Work out the finished part from the listing and answer in its coordinate system (mm). Give positions to 0.01 mm unless a question says otherwise; leave off trailing zeros. Order: outer loops, then holes, each group sorted by start corner. A loop starts at its lowest first (then second) coordinate and runs counter-clockwise, first axis right, second up. Notation, with made-up numbers: (77, 75.25) - (88, 75.25) arc R20 cw to (88, 113.25) - close; hole circle Ø1 at (-2, -12). An arc over 180 degrees is marked (long way). Write each question's results on one line, items separated by ' | '.
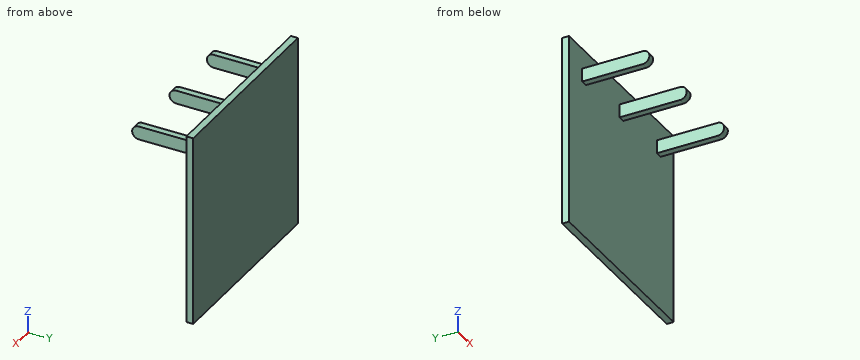
Autodesk Inventor part; units mm, degrees
ref_plane "pole_to_body_XY" through (0, 0.508, 0) normal (0, 1, 0) x (1, 0, 0)
ref_plane "pole_to_body_YZ" through (0, 0.508, 0) normal (1, 0, 0) x (0, 0, -1)
ref_plane "pole_to_body_ZX" through (0, 0.508, 0) normal (0, 0, -1) x (0, 1, 0)
sketch "Sketch_1" plane through (0, 0, 0) normal (0, 1, 0) x (-1, 0, 0)
  line L0 (7.112, -7.112) -> (7.112, 7.112)
  line L1 (7.112, 7.112) -> (-7.112, 7.112)
  line L2 (-7.112, 7.112) -> (-7.112, -7.112)
  line L3 (-7.112, -7.112) -> (7.112, -7.112)
extrude "Extrusion1" add sketch "Sketch_1" along normal blind 0.508
sketch "Sketch_10" plane through (-5.08, 0, 0) normal (1, 0, 0) x (0, 0, -1)
  arc A0 (-5.5753, -4.5085) -> (-5.08, -5.0038) centre (-5.08, -4.5085) ccw
  arc A1 (-5.08, -5.0038) -> (-4.5847, -4.5085) centre (-5.08, -4.5085) ccw
  line L0 (-4.5847, -4.5085) -> (-4.5847, 0.508)
  line L1 (-4.5847, 0.508) -> (-5.5753, 0.508)
  line L2 (-5.5753, 0.508) -> (-5.5753, -4.5085)
extrude "Extrusion2" add sketch "Sketch_10" along normal mid plane 0.508
sketch "Sketch_12" plane through (0, 0, 0) normal (1, 0, 0) x (0, 1, 0)
  arc A0 (-4.5085, 5.5753) -> (-5.0038, 5.08) centre (-4.5085, 5.08) ccw
  arc A1 (-5.0038, 5.08) -> (-4.5085, 4.5847) centre (-4.5085, 5.08) ccw
  line L0 (-4.5085, 4.5847) -> (0.508, 4.5847)
  line L1 (0.508, 4.5847) -> (0.508, 5.5753)
  line L2 (0.508, 5.5753) -> (-4.5085, 5.5753)
extrude "Extrusion3" add sketch "Sketch_12" along normal mid plane 0.508
sketch "Sketch_14" plane through (5.08, 0, 0) normal (1, 0, 0) x (0, 0, -1)
  arc A0 (-5.5753, -4.5085) -> (-5.08, -5.0038) centre (-5.08, -4.5085) ccw
  arc A1 (-5.08, -5.0038) -> (-4.5847, -4.5085) centre (-5.08, -4.5085) ccw
  line L0 (-4.5847, -4.5085) -> (-4.5847, 0.508)
  line L1 (-4.5847, 0.508) -> (-5.5753, 0.508)
  line L2 (-5.5753, 0.508) -> (-5.5753, -4.5085)
extrude "Extrusion4" add sketch "Sketch_14" along normal mid plane 0.508
ref_plane "pole_to_body_XY" through (0, 0.508, 0) normal (0, 1, 0) x (1, 0, 0)
ref_plane "pole_to_body_YZ" through (0, 0.508, 0) normal (1, 0, 0) x (0, 0, -1)
ref_plane "pole_to_body_ZX" through (0, 0.508, 0) normal (0, 0, -1) x (0, 1, 0)
properties part number "UB216SKG035D-NR"
1. A cutting plane is placed at A-A, the plane y = -2.45. Write down the section's boundary in (x, z), then the cut area to 3 significant figures.
Answer list:
outline: (-5.33, 4.58) - (-4.83, 4.58) - (-4.83, 5.58) - (-5.33, 5.58) - close; (-0.25, 4.58) - (0.25, 4.58) - (0.25, 5.58) - (-0.25, 5.58) - close; (4.83, 4.58) - (5.33, 4.58) - (5.33, 5.58) - (4.83, 5.58) - close | area: 1.51 mm^2
2. Given P1, Ø0.5, axis at y = -3.5, z = 5.5, coming from the +X side; P2, Ø0.8, axis at y = -2.5, z = 5, coming from the -X side; P3, Ø5, axis at x = -2.5, z = -5, coming from the -Y side; P4, Ø2, axis at x = 0.5, y = -0.5, coming from the -Z side, each flat-ended and moving along its own axis, determine where each tip first touches the part or whether it passes through.
Answer list:
P1: x = 5.33 | P2: x = -5.33 | P3: y = 0 | P4: z = -7.11
3. A cutting plane is placed at C-C, the plane x = -2. Write down the section's boundary in (y, z), then the cut area to 3 significant figures.
Answer list:
outline: (0, -7.11) - (0.51, -7.11) - (0.51, 7.11) - (0, 7.11) - close | area: 7.23 mm^2
4. Straight lines are drawn through the part: line 1 (Y direction, x = -0.25, z = -2); line 2 (Z direction, x = 5.25, y = -0.25). For each, find the intervals that lie inside material, in ascending order. Write a range as [from, to].
Answer list:
line 1: [0, 0.51] | line 2: [4.58, 5.58]
5. A cutting plane is placed at D-D, the plane z = -5.5. Write down the section's boundary in (x, y).
Answer list:
outline: (-7.11, 0) - (7.11, 0) - (7.11, 0.51) - (-7.11, 0.51) - close
6. A cutting plane is placed at B-B, the plane z = 5.08. Write down the section's boundary in (x, y).
Answer list:
outline: (-7.11, 0) - (-5.33, 0) - (-5.33, -5) - (-4.83, -5) - (-4.83, 0) - (-0.25, 0) - (-0.25, -5) - (0.25, -5) - (0.25, 0) - (4.83, 0) - (4.83, -5) - (5.33, -5) - (5.33, 0) - (7.11, 0) - (7.11, 0.51) - (-7.11, 0.51) - close
